Model file for the job. Use its own axes, mm. A direction names the side the tool comes from. Round coordinates to 2 decimals unless told otherwise and drop trailing zeros. Order: outer loops, then holes, each group sorted by start corner. A loop starts at its lowest first (then second) coordinate and runs counter-clockwise, first axis right, second up. Notation, with made-up numbers: (13, 75.25) - (51, 75.25) arc R22 cw to (51, 89.25) - close; hole circle Ø7 at (15.5, -2.5). An arc over 180 degrees is marked (long way). Use one line per item in the form item = value.
Autodesk Inventor part; units mm, degrees
ref_plane "YZ Plane" through (0, 0, 0) normal (1, 0, 0) x (0, 1, 0)
ref_plane "XZ Plane" through (0, 0, 0) normal (0, 1, 0) x (-1, 0, 0)
ref_plane "XY Plane" through (0, 0, 0) normal (0, 0, 1) x (1, 0, 0)
sketch "スケッチ1" plane through (0, 0, 0) normal (0, 0, 1) x (1, 0, 0)
  circle A0 centre (0, 0) radius 1.5
  dimension "d0" = 3
extrude "押し出し1" add sketch "スケッチ1" along normal blind 12
sketch "スケッチ2" plane through (0, 0, 0) normal (0, 0, -1) x (-1, 0, 0)
  circle A0 centre (0, 0) radius 3
  dimension "d3" = 6
extrude "押し出し2" add sketch "スケッチ2" against normal blind 2
thread "ねじ1"
chamfer "面取り1" distance 1.5 angle 45 1 edges at (3, 0, 2)
properties part number "ネジ皿m3,12" material "鋼、高強度、低合金"
(1) Slice it at D-D on z = 1.25. Give the cut face in (x, y), then the cut area to 3 significant figures.
Report:
outline = circle Ø4.5 at (0, 0)
area = 15.9 mm2
(2) Pin check, flat tips, straight feed: pin 1 (3 mm diameter, centred on x = -2.5, z = 10, fed in from +Y); pin 2 (2 mm diameter, centred on y = 1.5, z = 5, fed in from +X); pin 3 (1 mm diameter, centred on y = -0.5, z = 1.5, fed in from -X). Stop position of each tip, or through.
Report:
pin_1 = 1.12
pin_2 = 1.41
pin_3 = -2.46
(3) Probe probe 1 along X at (y, z) = (-0.1, 8); probe 2 along Y at (x, z) = (-0.8, 10.25); probe 3 along Z at (x, y) = (1.15, -1.6). List the from-to ranges inside material, lowest first. Write a range as [from, to].
Report:
probe_1 = [-1.5, 1.5]
probe_2 = [-1.27, 1.27]
probe_3 = [0, 1.53]
(4) Slice it at C-C on z = 8. Give the cut face in (x, y).
Report:
outline = circle Ø3 at (0, 0)
(5) Tool access for faces 1 (the face through (0, 0, 0)), 2 (the face through (-1.5, -0.07, 6.93)): list every direction of +Z, -Z, +X, -X, +Y, -Y with a clear straight run to the whole face (end or side of a thin tool).
Report:
face_1 = -Z, +X, -X, +Y, -Y
face_2 = +Z
